Read the model definition and answer for the solid it produces. Units are mm, in the model's axes. A direction names the side the tool comes from. Give positions to 0.01 mm unless a question says otherwise; leave off trailing zeros. Loops run counter-clockwise (first coordinate to the right, second up) from the corner with the lowest first, then second, coordinate; pieces in that order, holes last. Notation, with made-up numbers: (-3.75, 48) -> (40.25, 48) arc R28 ccw to (40.25, 86) -> close; hole circle Ø1 at (43.5, -27.5). An arc over 180 degrees is marked (long way). Write each question's results on one line, items separated by ' | '. Start each with the question number.
Item 1: Section C-C on y = 43 is taken. Write down the section's boundary in (x, z), and give its area (3 significant figures).
Item 2: Each of these flat-tipped pins is pushed along its axis until it touches: P1, Ø6.5, axis at y = 36, z = -8.5, coming from the +X side; P2, Ø7.5, axis at x = -13.716, y = 14.224, coming from the +Z side; P3, Ø4, axis at x = -22, y = 44, coming from the +Z side; P4, Ø1, axis at x = -54.5, z = 0, coming from the -Y side. Where does it stop, or does it pass through?
Item 3: Determine the mould class of faces 1 (the flat face through (-34.544, 38, -6)), 2 (the flat face through (-34, 76.2, 8)), 3 (the cylindrical face through (-20.06, 14.5, 11.33)) for opening direction X: +X half, -X half, draft (parallel to the pull), parting line (faces both ways), or undercut.
Item 4: Section A-A on z = 14 is taken. Write down the section's boundary in (x, y).
Item 5: Section D-D on x = -37 is taken. Write down the section's boundary in (y, z).
Item 6: Section B-B on y = 58 is taken. Write down the section's boundary in (x, z).
Item 7: Which of the six approach directions +Z, -Z, +X, -X, +Y, -Y give full straight-line access (tool end or side, diameter ignored) to faces 4 (the flat face through (-35, 43, 9.652)), 5 (the flat face through (-34.77, 53.763, 16.091)), 6 (the flat face through (-34.77, 27.86, 15.8))?
Item 8: Find the intervals of material crossed by line 1 (Z direction, x = -8.5, y = 26); line 2 (Z direction, x = -34, y = 48); line 3 (Y direction, x = -11, z = 6.5), in increasing order.
```python
from build123d import *

# Parameters (mm, degrees)
BOSS_EXTRUDE1_DEPTH = 76.2
CUT_EXTRUDE1_DEPTH  = 72.034516633
SKETCH5_R           = 6.35
CUT_EXTRUDE2_DEPTH  = 36.052


with BuildPart() as part:
    # Sketch1 → Boss-Extrude1 (new body)
    with BuildSketch(Plane(origin=(0, 0, 0), x_dir=(1, 0, 0), z_dir=(0, 1, 0))):
        Polygon((0, 0), (0, -22.352), (-68.58, -22.352), (-68.58, 12.7), (-34.544, 12.7), (-34.544, 0), align=None)
    extrude(amount=BOSS_EXTRUDE1_DEPTH)

    # Sketch2 → Cut-Extrude1 (cut, through all, along a direction that is not the sketch's normal)
    with BuildSketch(Plane.ZY.offset(68.58)):
        Polygon((22.352, 44.704), (9.652, 44.704), (9.652, 22.352), (22.352, 15.019651581), align=None)
    extrude(amount=-CUT_EXTRUDE1_DEPTH, dir=(-0.965925826, -0.258819045, 0), mode=Mode.SUBTRACT)

    # Sketch5 → Cut-Extrude2 (cut, through all)
    with BuildSketch(Plane.XY.offset(22.352)):
        with Locations((-54.864, 61.976)):
            Circle(SKETCH5_R)
        with Locations((-13.716, 14.224)):
            Circle(SKETCH5_R)
    extrude(amount=-CUT_EXTRUDE2_DEPTH, mode=Mode.SUBTRACT)


solid = part.part
```
Findings:
1) outline: (-68.58, -12.7) -> (-34.54, -12.7) -> (-34.54, 0) -> (0, 0) -> (0, 9.65) -> (-68.58, 9.65) -> close | area: 1,090 mm2
2) P1: x = -34.54 | P2: through | P3: z = 9.65 | P4: y = 0
3) face 1: +X half | face 2: draft | face 3: undercut
4) outline: (-68.58, 0) -> (0, 0) -> (0, 38.22) -> (-68.58, 19.84) -> close; (-68.58, 44.7) -> (0, 63.08) -> (0, 76.2) -> (-68.58, 76.2) -> close; hole circle Ø12.7 at (-54.86, 61.98); hole circle Ø12.7 at (-13.72, 14.22)
5) outline: (0, -12.7) -> (76.2, -12.7) -> (76.2, 22.35) -> (53.17, 22.35) -> (53.17, 9.65) -> (30.81, 9.65) -> (23.48, 22.35) -> (0, 22.35) -> close
6) outline: (-68.58, -12.7) -> (-59.82, -12.7) -> (-59.82, 22.35) -> (-68.58, 22.35) -> close; (-49.91, -12.7) -> (-34.54, -12.7) -> (-34.54, 0) -> (0, 0) -> (0, 9.65) -> (-18.96, 9.65) -> (-18.96, 22.35) -> (-49.91, 22.35) -> close
7) face 4: +Z | face 5: +Z, +X | face 6: +Z, -X
8) line 1: 0 to 22.35 | line 2: 0 to 9.65 | line 3: 0 to 8.48, 19.96 to 76.2
